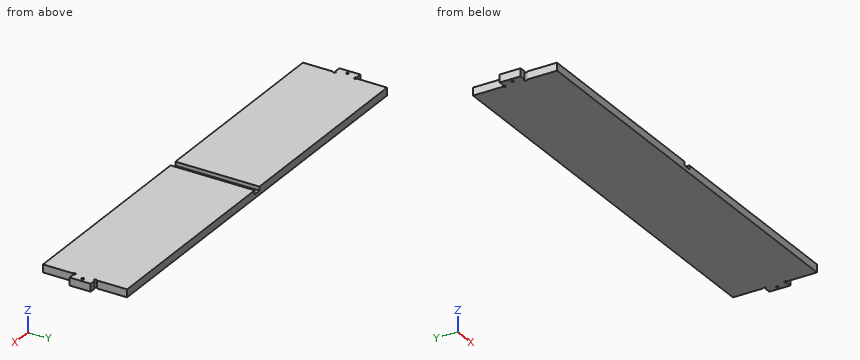
Autodesk Inventor part; units mm, degrees
ref_plane "YZ Plane" through (0, 0, 0) normal (1, 0, 0) x (0, 1, 0)
ref_plane "XZ Plane" through (0, 0, 0) normal (0, 1, 0) x (-1, 0, 0)
ref_plane "XY Plane" through (0, 0, 0) normal (0, 0, 1) x (1, 0, 0)
sketch "Sketch1" plane through (0, 0, 0) normal (0, 0, 1) x (1, 0, 0)
  line L0 (-48.4923, 85.7611) -> (-48.4923, 34.9611)
  line L1 (-48.4923, 34.9611) -> (-29.6963, 34.9611)
  line L2 (-29.6963, 34.9611) -> (-29.6963, -41.2389)
  line L3 (-29.6963, -41.2389) -> (986.3037, -41.2389)
  line L4 (986.3037, -41.2389) -> (986.3037, 34.9611)
  line L5 (986.3037, 34.9611) -> (1005.0997, 34.9611)
  line L6 (1005.0997, 34.9611) -> (1005.0997, 85.7611)
  line L7 (1005.0997, 85.7611) -> (986.3037, 85.7611)
  line L8 (986.3037, 85.7611) -> (986.3037, 161.9611)
  line L9 (986.3037, 161.9611) -> (-29.6963, 161.9611)
  line L10 (-48.4923, 85.7611) -> (-29.6963, 85.7611)
  line L11 (-29.6963, 85.7611) -> (-29.6963, 161.9611)
  point P0 (0, 0)
  dimension "d0" = 50.8
  dimension "d1" = 18.796
  dimension "d2" = 76.2
  dimension "d3" = 1016
  dimension "d4" = 76.2
  dimension "d5" = 18.796
  dimension "d6" = 50.8
  dimension "d7" = 76.2
  dimension "d8" = 18.796
extrude "Extrusion1" add sketch "Sketch1" along normal blind 18.796
sketch "Sketch2" plane through (0, 0, 18.796) normal (0, 0, 1) x (1, 0, 0)
  line L0 (-29.6963, 85.7611) -> (-48.4923, 85.7611)
  line L1 (-48.4923, 34.9611) -> (-29.6963, 34.9611)
  line L2 (1005.0997, 34.9611) -> (1005.0997, 85.7611)
  line L3 (-48.4923, 85.7611) -> (-48.4923, 34.9611)
  point P0 (0, 0)
  point P1 (-39.0943, 60.5407)
  point P2 (986.9445, 85.7611)
  point P3 (986.9445, 34.9611)
  point P4 (995.7017, 60.5407)
  dimension "d11" = 9.398
  dimension "d12" = 9.398
hole "Hole1" at (-29.6963, 85.7611, 18.796) at (-29.6963, 34.9611, 18.796) at (-39.0943, 60.5407, 18.796) at (986.9445, 85.7611, 18.796) at (986.9445, 34.9611, 18.796) at (995.7017, 60.5407, 18.796) direction (0, 0, -1) diameter 6.35 end through all
sketch "Sketch3" plane through (0, 0, 18.796) normal (0, 0, 1) x (1, 0, 0)
  line L0 (986.3037, 161.9611) -> (-29.6963, 161.9611)
  line L1 (478.3037, 161.9611) -> (478.3037, -41.2389)
  line L2 (-29.6963, -41.2389) -> (986.3037, -41.2389)
  line L3 (468.9057, 161.9611) -> (468.9057, -41.2389)
  line L4 (487.7017, 161.9611) -> (487.7017, -41.2389)
  line L5 (468.9057, 161.9611) -> (487.7017, 161.9611)
  line L6 (468.9057, -41.2389) -> (487.7017, -41.2389)
  point P0 (0, 0)
  dimension "d20" = 9.398
  dimension "d21" = 9.398
extrude "Extrusion2" cut sketch "Sketch3" against normal blind 9.398
properties part number "top" material "Wood (Birch)"
Source: CAD feature listing. Evaluate the final solid. Frame: model axes, mm. Round coordinates to 2 decimals unless told otherwise and drop trailing zeros. Loops run counter-clockwise (first coordinate to the right, second up) from the corner with the lowest first, then second, coordinate; pieces in that order, holes last.
(1) Material intervals for probe 1 along X at (y, z) = (59.5, 7.75); probe 2 along X at (y, z) = (35, 17); probe 3 along X at (y, z) = (122, 13), sorted ascending.
From the geometry:
probe 1: x = -48.49 to -42.09, -36.09 to 992.7, 998.7 to 1005.1
probe 2: x = -48.49 to -32.87, -26.52 to 468.91, 487.7 to 983.77, 990.12 to 1005.1
probe 3: x = -29.7 to 468.91, 487.7 to 986.3
(2) Section query A-A (z = 15.5). Give the number of separate pieces and of enclosed holes in the cut face, and give its area (3 significant figures).
From the geometry:
separate pieces: 2
enclosed holes: 2
area: 204,000 mm2
(3) Contact query for flat-ended pins moving along their axis: pin 1 Ø9.5 at (y, z) = (-6, 6.5) entering from +X; pin 2 Ø5.5 at (y, z) = (7, 10) entering from -X; pin 3 Ø7.5 at (x, z) = (1000, 7) entering from +Y; pin 4 Ø5.5 at (x, y) = (-29.7, 34.96) entering from -Z. Output: stop coordinate, or through.
From the geometry:
pin 1: stops at x = 986.3
pin 2: stops at x = -29.7
pin 3: stops at y = 85.76
pin 4: passes through
(4) Section query B-B (y = 0.5). Output: boundary loops of the cut face in (x, z).
From the geometry:
outline: (-29.7, 0) - (986.3, 0) - (986.3, 18.8) - (487.7, 18.8) - (487.7, 9.4) - (468.91, 9.4) - (468.91, 18.8) - (-29.7, 18.8) - close
